Can you work these out from the model? Positions are in its coordinate system, mm. A direction names the side the tool comes from. Give positions to 0.01 mm unless a question says otherwise; leave off trailing zeros. Write each loop counter-clockwise with the first axis right and the second up, starting at its lowest first coordinate (ties: lowest second). Pieces come first, ordered by that corner, then holes.
from build123d import *

# Parameters (mm, degrees)
F0_R     = 3.5
F1_DEPTH = 1
F2_R     = 4.25
F3_DEPTH = 6
F4_R     = 2.5
F5_DEPTH = 1.5
F7_R     = 2.5
F8_DEPTH = 6


# Not quite as in the source:
# - a fillet or chamfer that OpenCascade refuses, or shapes differently, is made with other operations: its cross-section is extruded or revolved along the edge and cut away or added


with BuildPart() as f1:
    # F0 (on Top) → F1 (new body)
    with BuildSketch(Plane.XY):
        Circle(F0_R)
    extrude(amount=F1_DEPTH)

    # F2 (on face) → F3 (join)
    with BuildSketch(Plane.XY.offset(1)):
        Circle(F2_R)
    extrude(amount=F3_DEPTH)

    # F4 (on face) → F5 (join)
    with BuildSketch(Plane.XY.offset(7)):
        Circle(F4_R)
    extrude(amount=F5_DEPTH)

    # F6: fillet of radius 1 on 2 edges, made by hand

    # F6_s1 → F6_t2 (revolve, cut)
    with BuildSketch(Plane.XZ):
        with BuildLine():
            ThreePointArc((4.25, 6), (3.9571067812, 6.7071067812), (3.25, 7))
            Line((3.25, 7), (4.25, 7))
            Line((4.25, 7), (4.25, 6))
        make_face()
    revolve(axis=Axis((0, 0, 7), (0, 0, 1)), mode=Mode.SUBTRACT)

    # F6_s3 → F6_t4 (revolve, cut)
    with BuildSketch(Plane.XZ):
        with BuildLine():
            ThreePointArc((4.25, 1.9682458366), (4.040569415, 1.3558734009), (3.5, 1))
            Line((3.5, 1), (4.25, 1))
            Line((4.25, 1), (4.25, 1.9682458366))
        make_face()
    revolve(axis=Axis((0, 0, 1), (0, 0, 1)), mode=Mode.SUBTRACT)

    # F7 (on face) → F8 (cut)
    with BuildSketch(Plane(origin=(0, 0, 0), x_dir=(1, 0, 0), z_dir=(0, 0, -1))):
        Circle(F7_R)
    extrude(amount=-F8_DEPTH, mode=Mode.SUBTRACT)


solid = f1.part
(1) Imagine slicing it at A-A, the plane y = 0. Write out the boundary of the cut face in (x, z), plus the area to 3 significant figures.
Returned:
outline: (-4.25, 1.97) arc R1 ccw to (-3.5, 1) - (-3.5, 0) - (-2.5, 0) - (-2.5, 6) - (2.5, 6) - (2.5, 0) - (3.5, 0) - (3.5, 1) arc R1 ccw to (4.25, 1.97) - (4.25, 6) arc R1 ccw to (3.25, 7) - (2.5, 7) - (2.5, 8.5) - (-2.5, 8.5) - (-2.5, 7) - (-3.25, 7) arc R1 ccw to (-4.25, 6) - close
area: 34.7 mm2
(2) If we mould it in two halves opening along Y, with no side actions, what happens to faces 1 (the face through (-0.54, 2.44, 2.96)), 2 (the face through (3.233, -1.341, 0.493)), 3 (the face through (2, -2, 0))? For each: +Y half, -Y half, draft (parallel to the pull), parting line (faces both ways), or undercut.
Returned:
face 1: undercut
face 2: parting line
face 3: draft
(3) Imagine slicing it at B-B, the plane z = 0.5. Write out the boundary of the cut face in (x, y), plus the area to 3 significant figures.
Returned:
outline: circle Ø7 at (0, 0); hole circle Ø5 at (0, 0)
area: 18.8 mm2
(4) Imagine slicing it at D-D, the plane z = 2.5. Write out the boundary of the cut face in (x, y), plus the area to 3 significant figures.
Returned:
outline: circle Ø8.5 at (0, 0); hole circle Ø5 at (0, 0)
area: 37.1 mm2
(5) If I drill on L1, parallel to Y at x = 0, z = 3; L2, parallel to Z at x = -3.25, y = 0.5; L3, parallel to Y at x = 0, z = 8.25, over which ranges is the centre line in solid material (lowest first)?
Returned:
L1: y = -4.25 to -2.5, 2.5 to 4.25
L2: z = 0 to 7
L3: y = -2.5 to 2.5
(6) For faces 4 (the face through (0, 0, 8.5)), 5 (the face through (-0.54, -2.44, 7.74)), 6 (the face through (0, 0, 6)), which set-ups out of +Z, -Z, +X, -X, +Y, -Y let a thin tool reach every point of the face, with its end or its side?
Returned:
face 4: +Z, +X, -X, +Y, -Y
face 5: +Z
face 6: -Z
(7) Will these pins go through, and if not, where does the flat tip stop? P1, Ø3, axis at x = -2.5, y = 0.5, coming from the +Z side; P2, Ø2.5, axis at x = 0, y = 0, coming from the -Z side; P3, Ø4, axis at x = -2.5, z = 6.5, coming from the +Y side.
Returned:
P1: stops at z = 8.5
P2: stops at z = 6
P3: stops at y = 4.21
